```python
from build123d import *

# Parameters (mm, degrees)
SKETCH1_R          = 18
BASE_EXTRUDE_DEPTH = 361.5
SKETCH2_R          = 62.5
PISTON_DEPTH       = 5
FLATS_DEPTH        = 373.148827756
FLATS_DEPTH_BACK   = 373.148827756


with BuildPart() as part:
    # Sketch1 → Base-Extrude (new body)
    with BuildSketch(Plane.XY):
        Circle(SKETCH1_R)
    extrude(amount=BASE_EXTRUDE_DEPTH)

    # Sketch2 → Piston (add)
    with BuildSketch(Plane(origin=(0, 0, 0), x_dir=(-1, 0, 0), z_dir=(0, 0, -1))):
        Circle(SKETCH2_R)
    extrude(amount=-PISTON_DEPTH)

    # Sketch3 → Thread (revolve, cut)
    with BuildSketch(Plane(origin=(0, 0, 0), x_dir=(0, 0, -1), z_dir=(1, 0, 0)), mode=Mode.PRIVATE) as thread_sk:
        Polygon((-361.5, 18), (-361.5, 13), (-359.5, 15), (-311.5, 15), (-308.5, 18), align=None)
    revolve(thread_sk.sketch.rotate(Axis((0, 0, 0), (0, 0, 1)), 90), axis=Axis((0, 0, 0), (0, 0, 1)), mode=Mode.SUBTRACT)

    # Sketch4 → Flats (cut, two sides: drawn at the far end of the back side and taken through both)
    with BuildSketch(Plane(origin=(0, 0, 0), x_dir=(1, 0, 0), z_dir=(0, 1, 0)).offset(-FLATS_DEPTH_BACK)):
        Polygon((18, -294), (15.5, -296.5), (15.5, -361.5), (18, -361.5), align=None)
        Polygon((-18, -361.5), (-18, -294), (-15.5, -296.5), (-15.5, -361.5), align=None)
    extrude(amount=FLATS_DEPTH + FLATS_DEPTH_BACK, mode=Mode.SUBTRACT)


solid = part.part
```
Build history of the part. All positions in model axes, mm. A direction names the side the tool comes from. Coordinates: 2 decimals unless noted, no trailing zeros. Order: outer loops, then holes, each group sorted by start corner. A loop starts at its lowest first (then second) coordinate and runs counter-clockwise, first axis right, second up. Notation, with made-up numbers: M 4.5,69 L 54.5,69 A24 ccw 54.5,99 Z; hole C -24.75,31.25 d4. An arc over 180 degrees is marked long. One line per question, with ' | ' between items. Start each with the question number.
1. Cut at B-B (x = 0). Write the cut outline in (y, z).
2. Cut at C-C (z = 192). Write the cut outline in (x, y), plus the area to 3 significant figures.
3. Wall check: line 1 along Z through (x, y) = (-48, 4.5); line 2 along Y through (x, z) = (-15.5, 125.5); line 3 along X through (y, z) = (-16, 160). Give the ranges that are in metal, low to high. Write a range as [from, to].
4. Cut at D-D (y = 50). Write the cut outline in (x, z), plus the area to 3 significant figures.
5. Flat gauge pins, fed straight in: P1, Ø7, axis at y = 1.5, z = 307, coming from the +X side; P2, Ø10, axis at x = 42, y = -39, coming from the -Z side; P3, Ø1.5, axis at y = 9, z = 325, coming from the +X side; P4, Ø3, axis at x = -9.5, z = 236.5, coming from the +Y side. Where does each tip first touch, or does it go through?
6. Tool access for faces 1 (the face through (1, 1, 0)), 2 (the face through (15.5, 0, 304)), 3 (the face through (-13, -13, 5)), 4 (the face through (62.44, 2.75, 2.46)), 5 (the face through (-15.5, 0, 304)): list every direction of +Z, -Z, +X, -X, +Y, -Y with a clear straight run to the whole face (end or side of a thin tool).
7. Cut at A-A (y = 0). Write the cut outline in (x, z), plus the area to 3 significant figures.
The answers:
1) outline: M -62.5,0 L 62.5,0 L 62.5,5 L 18,5 L 18,308.5 L 15,311.5 L 15,359.5 L 13,361.5 L -13,361.5 L -15,359.5 L -15,311.5 L -18,308.5 L -18,5 L -62.5,5 Z
2) outline: C 0,0 d36 | area: 1,020 mm2
3) line 1: z = [0, 5] | line 2: y = [-9.15, 9.15] | line 3: x = [-8.25, 8.25]
4) outline: M -37.5,0 L 37.5,0 L 37.5,5 L -37.5,5 Z | area: 375 mm2
5) P1: stops at x = 15.5 | P2: stops at z = 0 | P3: stops at x = 12.53 | P4: stops at y = 16.12
6) face 1: -Z, +X, -X, +Y, -Y | face 2: +Z, +X, +Y, -Y | face 3: +Z | face 4: +Z, -Z | face 5: +Z, -X, +Y, -Y
7) outline: M -62.5,0 L 62.5,0 L 62.5,5 L 18,5 L 18,294 L 15.5,296.5 L 15.5,311 L 15,311.5 L 15,359.5 L 13,361.5 L -13,361.5 L -15,359.5 L -15,311.5 L -15.5,311 L -15.5,296.5 L -18,294 L -18,5 L -62.5,5 Z | area: 13,100 mm2
